Verification items for the finished model (mm, model axes). A direction names the side the tool comes from. Coordinates: 2 decimals unless noted, no trailing zeros. Loops run counter-clockwise (first coordinate to the right, second up) from the corner with the lowest first, then second, coordinate; pieces in that order, holes last. Notation, with made-up numbers: (67.5, -36.5) - (72.5, -36.5) arc R32 cw to (72.5, -10.5) - close; hole circle Ø5 at (-30.5, 32.5). An arc over 180 degrees is marked (long way). One line per item, written item: value. Start each with the question number.
(1) Section check B-B (x = 0). Record the boundary of the cut face in (y, z), plus the area to 3 significant figures.
(2) Section check C-C (y = -2.25). Record the boundary of the cut face in (x, z), plus the area to 3 significant figures.
(3) Thickness scan on probe 1 along Z at (x, y) = (0, 3.5); probe 2 along Z at (x, y) = (0, -2.75); probe 3 along X at (y, z) = (-3.25, 2.5). Record the ranges inside material, lowest first. Write a range as [from, to].
(4) Draft check along X on faces 1 (the face through (-1, -5, -20)), 2 (the face through (-12.5, 0, 26)), 3 (the face through (0, 0, 15.3)). Enter one of: +X half, -X half, draft (parallel to the pull), parting line (faces both ways), or undercut.
(5) Section check D-D (z = -3). Record the boundary of the cut face in (x, y).
(6) Section check A-A (z = 6.5). Record the boundary of the cut face in (x, y).
(7) Gauge pin test, flat ends, axial feed: P1, Ø10, axis at y = -2, z = 1.5, coming from the -X side; P2, Ø6.5, axis at x = 4.5, z = 28, coming from the -Y side; P3, Ø4, axis at y = -2.5, z = 9.5, coming from the +X side. Record the tip position at first contact, or that the pin passes through.
(8) Set-up check for faces 4 (the face through (16, 0, 20)), 5 (the face through (15.3, 0, 12)), 6 (the face through (-2.38, -1.05, 21.26)), 7 (the face through (-16, 0, 20)): record each of +Z, -Z, +X, -X, +Y, -Y from which the full face is reachable in a straight line by a thin tool's end or side.
Solid Edge part; units mm, degrees
sketch "Sketch1" plane through (0, 0, 0) normal (0, -1, 0) x (1, 0, 0)
  line L0 (-20, -20) -> (20, -20)
  line L1 (20, -20) -> (20, 20)
  line L2 (20, 20) -> (-20, 20)
  line L3 (-20, 20) -> (-20, -20)
extrude "Protrusion1" add sketch "Sketch1" along normal mid plane 9
sketch "Sketch2" plane through (0, -4.5, 0) normal (0, -1, 0) x (1, 0, 0)
  line L0 (-15.3, -15.3) -> (15.3, -15.3)
  line L1 (15.3, -15.3) -> (15.3, -9)
  line L2 (10.3, -4) -> (15.3, -9)
  line L3 (10.3, 4) -> (10.3, -4)
  line L4 (10.3, 4) -> (15.3, 9)
  line L5 (15.3, 9) -> (15.3, 15.3)
  line L6 (15.3, 15.3) -> (-15.3, 15.3)
  line L7 (-15.3, 15.3) -> (-15.3, 9)
  line L8 (-10.3, 4) -> (-15.3, 9)
  line L9 (-10.3, 4) -> (-10.3, -4)
  line L10 (-10.3, -4) -> (-15.3, -9)
  line L11 (-15.3, -9) -> (-15.3, -15.3)
extrude "ExtrudedCutout_1" cut sketch "Sketch2" against normal blind 161.5
sketch "Sketch3" plane through (0, -4.5, 2.35) normal (0, -1, 0) x (1, 0, 0)
  line L0 (-12.5, 29.65) -> (-12.5, 17.65)
  line L1 (-12.5, 17.65) -> (12.5, 17.65)
  line L2 (12.5, 29.65) -> (12.5, 17.65)
  arc A0 (12.5, 29.65) -> (-12.5, 29.65) centre (0, 29.65) ccw
extrude "Protrusion2" add sketch "Sketch3" against normal blind 7
sketch "Sketch4" plane through (0, -4.5, 14.6) normal (0, -1, 0) x (1, 0, 0)
  circle A0 centre (0, 17.4) radius 11
extrude "ExtrudedCutout_2" cut sketch "Sketch4" against normal blind 39
sketch "Sketch5" plane through (0, 2.5, 32.25) normal (0, 1, 0) x (0, 0, -1)
  line L0 (0.25, -12.5) -> (12.25, -12.5)
  line L1 (12.25, -12.5) -> (12.25, 12.5)
  line L2 (12.25, 12.5) -> (0.25, 12.5)
  arc A0 (0.25, 12.5) -> (0.25, -12.5) centre (0.25, 0) ccw
extrude "ExtrudedProtrusion_4" add sketch "Sketch5" along normal blind 2
sketch "Sketch6" plane through (0, 4.5, 14.6) normal (0, 1, 0) x (0, 0, -1)
  circle A0 centre (-17.4, 0) radius 4.5
extrude "ExtrudedCutout_3" cut sketch "Sketch6" against normal blind 37
sketch "Sketch7" plane through (0, 0, -20) normal (0, 0, -1) x (1, 0, 0)
  line L0 (40, -4.5) -> (-40, -4.5)
  line L1 (-40, -4.5) -> (-40, 15.5)
  line L2 (-40, 15.5) -> (40, 15.5)
  line L3 (40, 15.5) -> (40, -4.5)
  dimension "D1" = 40
extrude "Protrusion3" add sketch "Sketch7" against normal blind 4.7
fillet "Round_2" radius 10 4 edges at (-40, -15.5, -17.65) (40, 4.5, -17.65) (40, -15.5, -17.65) (-40, 4.5, -17.65)
Responses:
1. outline: (-15.5, -20) - (4.5, -20) - (4.5, -15.3) - (-15.5, -15.3) - close; (-4.5, 15.3) - (4.5, 15.3) - (4.5, 27.5) - (2.5, 27.5) - (2.5, 21) - (-4.5, 21) - close; (-4.5, 43) - (2.5, 43) - (2.5, 36.5) - (4.5, 36.5) - (4.5, 44.5) - (-4.5, 44.5) - close
1. area: 185 mm²
2. outline: (-39.46, -20) - (39.46, -20) - (39.46, -15.3) - (20, -15.3) - (20, 20) - (12.5, 20) - (12.5, 32) arc R12.5 ccw to (-12.5, 32) - (-12.5, 20) - (-20, 20) - (-20, -15.3) - (-39.46, -15.3) - close; hole (-15.3, -15.3) - (15.3, -15.3) - (15.3, -9) - (10.3, -4) - (10.3, 4) - (15.3, 9) - (15.3, 15.3) - (-15.3, 15.3) - (-15.3, 9) - (-10.3, 4) - (-10.3, -4) - (-15.3, -9) - close; hole circle Ø22 at (0, 32)
2. area: 1,140 mm²
3. probe 1: z = [-20, -15.3], [15.3, 27.5], [36.5, 44.5]
3. probe 2: z = [-20, -15.3], [15.3, 21], [43, 44.5]
3. probe 3: x = [-20, -10.3], [10.3, 20]
4. face 1: draft
4. face 2: -X half
4. face 3: undercut
5. outline: (-20, -4.5) - (-10.3, -4.5) - (-10.3, 4.5) - (-20, 4.5) - close; (10.3, -4.5) - (20, -4.5) - (20, 4.5) - (10.3, 4.5) - close
6. outline: (-20, -4.5) - (-12.8, -4.5) - (-12.8, 4.5) - (-20, 4.5) - close; (12.8, -4.5) - (20, -4.5) - (20, 4.5) - (12.8, 4.5) - close
7. P1: stops at x = -20
7. P2: stops at y = 2.5
7. P3: stops at x = 20
8. face 4: +Z, +X, +Y, -Y
8. face 5: +Y, -Y
8. face 6: -Y
8. face 7: +Z, -X, +Y, -Y
